```python
from build123d import *

# Parameters (mm, degrees)
SKETCH1_R           = 21
SKETCH1_R_2         = 8.1875
BOSS_EXTRUDE1_DEPTH = 37.3
SKETCH2_R           = 24
SKETCH2_R_2         = 21
BOSS_EXTRUDE2_DEPTH = 27.3
SKETCH3_R           = 12.75
CUT_EXTRUDE1_DEPTH  = 6.1
SKETCH4_R           = 11.5
CUT_EXTRUDE2_DEPTH  = 2
MOVE_FACE2_BY       = 5
SKETCH6_R           = 24
SKETCH6_R_2         = 20
CUT_EXTRUDE3_DEPTH  = 20
CHAMFER1_SIZE2      = 4
CHAMFER1_SIZE       = 8
CHAMFER2_SIZE       = 1.5
CHAMFER3_SIZE       = 4


with BuildPart() as part:
    # Sketch1 → Boss-Extrude1 (new body)
    with BuildSketch(Plane.XY):
        Circle(SKETCH1_R)
        Circle(SKETCH1_R_2, mode=Mode.SUBTRACT)
    extrude(amount=BOSS_EXTRUDE1_DEPTH)

    # Sketch2 → Boss-Extrude2 (add)
    with BuildSketch(Plane(origin=(0, 0, 0), x_dir=(-1, 0, 0), z_dir=(0, 0, -1))):
        Circle(SKETCH2_R)
        with Locations(Location((0, 0, 0), (0, 0, 180))):
            Circle(SKETCH2_R_2, mode=Mode.SUBTRACT)
    extrude(amount=-BOSS_EXTRUDE2_DEPTH)

    # Sketch3 → Cut-Extrude1 (cut)
    with BuildSketch(Plane.XY.offset(37.3)):
        Circle(SKETCH3_R)
    extrude(amount=-CUT_EXTRUDE1_DEPTH, mode=Mode.SUBTRACT)

    # Sketch4 → Cut-Extrude2 (cut)
    with BuildSketch(Plane(origin=(0, 0, 0), x_dir=(-1, 0, 0), z_dir=(0, 0, -1))):
        Circle(SKETCH4_R)
    extrude(amount=-CUT_EXTRUDE2_DEPTH, mode=Mode.SUBTRACT)

    # Move Face2: a curved face moved inward by 5.0
    add(Solid.thicken(part.faces().sort_by_distance((-21, 0, 32.3))[0], -MOVE_FACE2_BY), mode=Mode.SUBTRACT)

    # Sketch6 → Cut-Extrude3 (cut)
    with BuildSketch(Plane(origin=(0, 0, 0), x_dir=(-1, 0, 0), z_dir=(0, 0, -1))):
        Circle(SKETCH6_R)
        Circle(SKETCH6_R_2, mode=Mode.SUBTRACT)
    extrude(amount=-CUT_EXTRUDE3_DEPTH, mode=Mode.SUBTRACT)

    # Chamfer1
    chamfer1_edges = [part.edges().sort_by_distance(p)[0] for p in [
        (24, 0, 27.3),
    ]]
    chamfer1_side = [part.faces().sort_by_distance(p)[0] for p in [
        (23.92, 0, 27.3),
    ]]
    chamfer(chamfer1_edges, length=CHAMFER1_SIZE - 0.0001, length2=CHAMFER1_SIZE2 - 0.0001, reference=chamfer1_side[0])  # a hair under: the kernel refuses the full size

    # Chamfer2
    chamfer2_edges = [part.edges().sort_by_distance(p)[0] for p in [
        (-8.1875, 0, 31.2),
        (-8.1875, 0, 2),
    ]]
    chamfer(chamfer2_edges, length=CHAMFER2_SIZE)

    # Fillet1: read off the stored shape, not the designer's step
    # Fillet1 outline → Fillet1 (revolve, cut)
    with BuildSketch(Plane.XZ):
        with BuildLine():
            ThreePointArc((23.170820393, 23.714589803), (23.775976213, 23.161545685), (24, 22.372949017))
            Line((24, 22.372949017), (24, 23.714589803))
            Line((24, 23.714589803), (23.170820393, 23.714589803))
        make_face()
    revolve(axis=Axis((0, 0, 0), (0, 0, 1)), mode=Mode.SUBTRACT)

    # Fillet1 2 outline → Fillet1 2 (revolve)
    with BuildSketch(Plane.XZ):
        with BuildLine():
            Line((16, 26.885410197), (16.829179607, 26.885410197))
            ThreePointArc((16.829179607, 26.885410197), (16.224023787, 27.438454315), (16, 28.227050983))
            Line((16, 28.227050983), (16, 26.885410197))
        make_face()
    revolve(axis=Axis((0, 0, 0), (0, 0, 1)))

    # Chamfer3
    chamfer3_edges = [part.edges().sort_by_distance(p)[0] for p in [
        (20, 0, 20),
    ]]
    chamfer(chamfer3_edges, length=CHAMFER3_SIZE - 0.0001)  # a hair under: the kernel refuses the full size

    # Fillet3: read off the stored shape, not the designer's step
    # Fillet3 outline → Fillet3 (revolve, cut)
    with BuildSketch(Plane.XZ):
        with BuildLine():
            ThreePointArc((24, 20.621320344), (23.885819299, 20.047295195), (23.560660172, 19.560660172))
            Line((23.560660172, 19.560660172), (24, 19.560660172))
            Line((24, 19.560660172), (24, 20.621320344))
        make_face()
    revolve(axis=Axis((0, 0, 0), (0, 0, 1)), mode=Mode.SUBTRACT)

    # Fillet3 2 outline → Fillet3 2 (revolve)
    with BuildSketch(Plane.XZ):
        with BuildLine():
            ThreePointArc((20, 15.378679656), (20.114180701, 15.952704805), (20.439339828, 16.439339828))
            Line((20.439339828, 16.439339828), (20, 16.439339828))
            Line((20, 16.439339828), (20, 15.378679656))
        make_face()
    revolve(axis=Axis((0, 0, 0), (0, 0, 1)))


solid = part.part
```
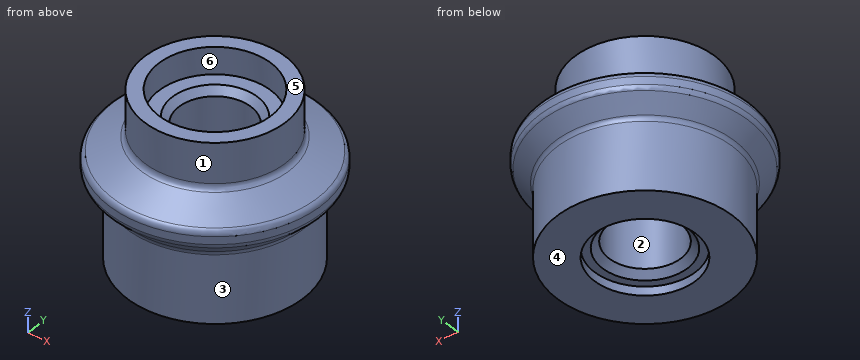
Model file for the job. Use its own axes, mm. Face numbers are marked on the shaded views. A direction names the side the tool comes from. Round coordinates to 2 decimals unless told otherwise and drop trailing zeros. Write each loop counter-clockwise with the first axis right and the second up, starting at its lowest first coordinate (ties: lowest second). Pieces come first, ordered by that corner, then holes. Notation, with made-up numbers: (70, 11) -> (75, 11) arc R21 ccw to (75, 23) -> close; hole circle Ø8 at (30, 35). An arc over 180 degrees is marked (long way). Answer as CSV lines item,"result".
1. Slice it at B-B, the plane z = 32. List the corners of the cut face in (x, y), plus the area to 3 significant figures.
Resolved:
outline,"circle Ø32 at (0, 0); hole circle Ø25.5 at (0, 0)"
area,"294 mm²"
2. Mould opens along Z. For the marked faces 4, 5 and 6 say: +Z half, -Z half, draft (parallel to the pull), parting line (faces both ways), or undercut.
Resolved:
face 4,"-Z half"
face 5,"+Z half"
face 6,"draft"
3. Tool access for the marked faces 1, 2 and 3: list every direction of +Z, -Z, +X, -X, +Y, -Y with a clear straight run to the whole face (end or side of a thin tool).
Resolved:
face 1,"+Z"
face 2,"+Z, -Z"
face 3,"-Z"
4. Drill centre lines: line 1 (Y direction, x = 0, z = 34); line 2 (Y direction, x = 0, z = 13.5); line 3 (X direction, y = 0.5, z = 33). Where is each one in solid material? Low to high.
Resolved:
line 1,"-16 to -12.75, 12.75 to 16"
line 2,"-20 to -8.19, 8.19 to 20"
line 3,"-15.99 to -12.74, 12.74 to 15.99"
5. Slice it at A-A, the plane z = 21.5. List the corners of the cut face in (x, y) (1 decimal), plus the area to 3 significant figures.
Resolved:
outline,"circle Ø48 at (0, 0); hole circle Ø16.4 at (0, 0)"
area,"1,600 mm²"
6. Pin check, flat tips, straight feed: pin 1 Ø4 at (x, z) = (-10, 24.5) entering from +Y; pin 2 Ø11.5 at (x, y) = (-0.5, 2) entering from -Z; pin 3 Ø4 at (y, z) = (9.5, 16.5) entering from +X; pin 4 Ø3 at (x, z) = (-7.5, 21.5) entering from -Y. Stop position of each tip, or through.
Resolved:
pin 1,"y = 22.23"
pin 2,"through"
pin 3,"x = 20.57"
pin 4,"y = -23.24"
